from build123d import *

# Parameters (mm, degrees)
BOSS_EXTRU_1_DEPTH                                 = 12
TROU_TARAUD_M61_D                                  = 5
TROU_TARAUD_M62_D                                  = 5
CHAMBRAGE_POUR_VIS_T_TE_HEXAGONALE_M51_D           = 5.5
CHAMBRAGE_POUR_VIS_T_TE_HEXAGONALE_M51_CBORE_D     = 10
CHAMBRAGE_POUR_VIS_T_TE_HEXAGONALE_M51_CBORE_DEPTH = 5
ESQUISSE11_R                                       = 7
ENL_V_MAT_EXTRU_1_DEPTH                            = 13
R_P_TITION_CIRCULAIRE1_COUNT                       = 3
ESQUISSE12_R                                       = 23.25
ENL_V_MAT_EXTRU_2_DEPTH                            = 1
ENL_V_MAT_EXTRU_4_DEPTH                            = 13
ENL_V_MAT_EXTRU_5_DEPTH                            = 13
ENL_V_MAT_EXTRU_6_DEPTH                            = 9


with BuildPart() as part:
    # Esquisse1 → Boss.-Extru.1 (new body)
    with BuildSketch(Plane.XY):
        with BuildLine():
            Line((270, 17.320508076), (-120, 242.48711306))
            ThreePointArc((-120, 242.48711306), (-140, 242.48711306), (-150, 225.166604984))
            Line((-150, 225.166604984), (-150, -225.166604984))
            ThreePointArc((-150, -225.166604984), (-140, -242.48711306), (-120, -242.48711306))
            Line((-120, -242.48711306), (270, -17.320508076))
            ThreePointArc((270, -17.320508076), (280, 0), (270, 17.320508076))
        make_face()
    extrude(amount=BOSS_EXTRU_1_DEPTH)

    # Trou taraudé M61 (through all)
    with Locations(Plane(origin=(0, 0, 0), x_dir=(1, 0, 0), z_dir=(0, 0, -1))):
        with Locations((260, 0)):
            Hole(TROU_TARAUD_M61_D / 2)

    # Trou taraudé M62 (through all)
    with Locations(Plane.XY.offset(12)):
        with Locations((-130.266309147, -225.083745367), (-130, 225.166604984)):
            Hole(TROU_TARAUD_M62_D / 2)

    # Chambrage pour vis à tête hexagonale M51 (through all)
    with Locations(Plane.XY.offset(12)):
        with Locations((19.5, 0)):
            chambrage_pour_vis_t_te_hexagonale_m51 = CounterBoreHole(CHAMBRAGE_POUR_VIS_T_TE_HEXAGONALE_M51_D / 2, CHAMBRAGE_POUR_VIS_T_TE_HEXAGONALE_M51_CBORE_D / 2, CHAMBRAGE_POUR_VIS_T_TE_HEXAGONALE_M51_CBORE_DEPTH)

    # Esquisse11 → Enlèv. mat.-Extru.1 (cut, through all)
    with BuildSketch(Plane.XY.offset(12)):
        Circle(ESQUISSE11_R)
    extrude(amount=-ENL_V_MAT_EXTRU_1_DEPTH, mode=Mode.SUBTRACT)

    # Répétition circulaire1: Chambrage pour vis à tête hexagonale M51 ×3 about axis
    r_p_tition_circulaire1_axis = Axis((0, 0, 0), (0, 0, 1))
    for i in range(1, R_P_TITION_CIRCULAIRE1_COUNT):
        add(chambrage_pour_vis_t_te_hexagonale_m51.rotate(r_p_tition_circulaire1_axis, i * 360 / R_P_TITION_CIRCULAIRE1_COUNT), mode=Mode.SUBTRACT)

    # Esquisse12 → Enlèv. mat.-Extru.2 (cut)
    with BuildSketch(Plane(origin=(0, 0, 0), x_dir=(-1, 0, 0), z_dir=(0, 0, -1))):
        Circle(ESQUISSE12_R)
    extrude(amount=-ENL_V_MAT_EXTRU_2_DEPTH, mode=Mode.SUBTRACT)

    # Esquisse15 → Enlèv. mat.-Extru.4 (cut, through all)
    with BuildSketch(Plane(origin=(0, 0, 0), x_dir=(-1, 0, 0), z_dir=(0, 0, -1))):
        with BuildLine():
            Line((117, 137.502524439), (117, 62.497475561))
            ThreePointArc((117, 62.497475561), (95, 40.497475561), (73, 62.497475561))
            Line((73, 62.497475561), (73, 137.502524439))
            ThreePointArc((73, 137.502524439), (95, 159.502524439), (117, 137.502524439))
        make_face()
    extrude(amount=-ENL_V_MAT_EXTRU_4_DEPTH, mode=Mode.SUBTRACT)

    # Esquisse16 → Enlèv. mat.-Extru.5 (cut, through all)
    with BuildSketch(Plane.XY.offset(12)):
        with BuildLine():
            Line((-139.9, 140), (-139.9, 60))
            ThreePointArc((-139.9, 60), (-142.5, 57.4), (-145.1, 60))
            Line((-145.1, 60), (-145.1, 140))
            ThreePointArc((-145.1, 140), (-142.5, 142.6), (-139.9, 140))
        make_face()
    extrude(amount=-ENL_V_MAT_EXTRU_5_DEPTH, mode=Mode.SUBTRACT)

    # Esquisse17 → Enlèv. mat.-Extru.6 (cut)
    with BuildSketch(Plane.XY.offset(12)):
        with BuildLine():
            Line((-138, 140), (-138, 60))
            ThreePointArc((-138, 60), (-142.5, 55.5), (-147, 60))
            Line((-147, 60), (-147, 140))
            ThreePointArc((-147, 140), (-142.5, 144.5), (-138, 140))
        make_face()
    extrude(amount=-ENL_V_MAT_EXTRU_6_DEPTH, mode=Mode.SUBTRACT)


solid = part.part
CAD build for the part. Positions are in the model's coordinates, mm. A direction names the side the tool comes from. Coordinates: 2 decimals unless noted, no trailing zeros. Order: outer loops, then holes, each group sorted by start corner. A loop starts at its lowest first (then second) coordinate and runs counter-clockwise, first axis right, second up. Notation, with made-up numbers: (-37.75, 33.25) -> (-32.75, 33.25) arc R11 ccw to (-32.75, 44.25) -> close; hole circle Ø5 at (21.5, 10). An arc over 180 degrees is marked (long way). Answer in a Markdown table with one row per item.
1) Flat gauge pins, fed straight in: P1, Ø1, axis at x = 163, z = 5, coming from the +Y side; P2, Ø3, axis at x = -130, y = 225.17, coming from the +Z side; P3, Ø2, axis at x = 34, z = 5, coming from the +Y side; P4, Ø23, axis at x = -1, y = 6.5, coming from the -Z side. Where does each tip first touch, or does it go through?
Check values:
| item | result |
|---|---|
| P1 | y = 79.39 |
| P2 | through |
| P3 | y = 154.15 |
| P4 | z = 1 |
2) Band-saw the part on A-A (x = -95). List the corners of the cut face in (y, z).
Check values:
| item | result |
|---|---|
| outline | (-228.05, 0) -> (40.5, 0) -> (40.5, 12) -> (-228.05, 12) -> close; (159.5, 0) -> (228.05, 0) -> (228.05, 12) -> (159.5, 12) -> close |
3) Band-saw the part on D-D (x = 77.5). List the corners of the cut face in (y, z).
Check values:
| item | result |
|---|---|
| outline | (-128.46, 0) -> (128.46, 0) -> (128.46, 12) -> (-128.46, 12) -> close |
4) Band-saw the part on C-C (y = -111). List the corners of the cut face in (x, z).
Check values:
| item | result |
|---|---|
| outline | (-150, 0) -> (107.74, 0) -> (107.74, 12) -> (-150, 12) -> close |
5) Band-saw the part on B-B (y = 102.5). List the corners of the cut face in (x, z).
Check values:
| item | result |
|---|---|
| outline | (-150, 0) -> (-145.1, 0) -> (-145.1, 3) -> (-147, 3) -> (-147, 12) -> (-150, 12) -> close; (-139.9, 0) -> (-117, 0) -> (-117, 12) -> (-138, 12) -> (-138, 3) -> (-139.9, 3) -> close; (-73, 0) -> (122.46, 0) -> (122.46, 12) -> (-73, 12) -> close |
6) Mould opens along X. For faces 6 (the face through (-9, 20, 7)), 7 (the face through (-140.25, -242.34, 5.92)), 8 (the face through (280, 0, 6)) say: pulls with the +X half, pulls with the -X half, needs draft (parallel to the pull), parting line crosses it, or undercut.
Check values:
| item | result |
|---|---|
| face 6 | undercut |
| face 7 | parting line crosses it |
| face 8 | pulls with the +X half |
7) Drill centre lines: line 1 (Y direction, x = -130, z = 5.5); line 2 (X direction, y = 102, z = 2.5); line 3 (Y direction, x = -9.75, z = 5.65). Where is each one in solid material? Low to high.
Check values:
| item | result |
|---|---|
| line 1 | -245.17 to -227.57, -222.6 to 222.67, 227.67 to 245.17 |
| line 2 | -150 to -145.1, -139.9 to -117, -73 to 123.33 |
| line 3 | -178.83 to -19.64, -14.14 to 14.14, 19.64 to 178.83 |
8) Which spindle directions (+Z, -Z, +X, -X, +Y, -Y) get a long thin tool onto all of the face, cutting with end or side? Do faces 1 (the face through (77.73, 128.328, 5.916)), 2 (the face through (-95.484, 40.503, 5.916)), 3 (the face through (14, 3, 12)), 4 (the face through (-22.176, 6.984, 0.493)), 5 (the face through (-4.98, 18.39, 9.54)). Say none if no direction does.
Check values:
| item | result |
|---|---|
| face 1 | +Z, -Z, +X, +Y |
| face 2 | +Z, -Z |
| face 3 | +Z, +X, -X, +Y, -Y |
| face 4 | -Z |
| face 5 | +Z |
